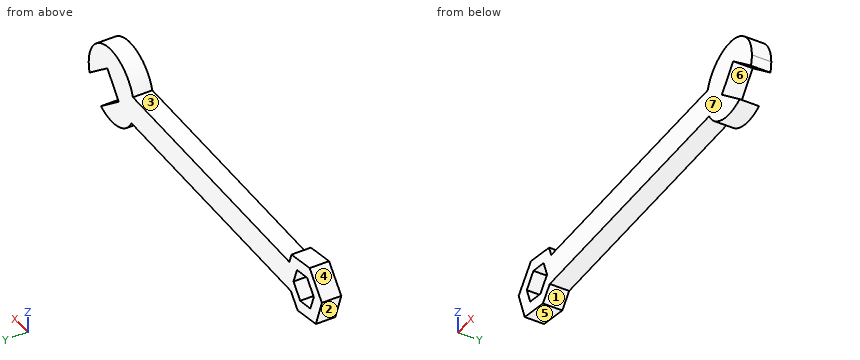
```python
from build123d import *

# Parameters (mm, degrees)
F1_DEPTH = 6.35


with BuildPart() as f1:
    # F0 (on Front) → F1 (new body)
    with BuildSketch(Plane.XZ):
        with BuildLine():
            Line((-19.535648028, 41.1698554981), (69.6690051493, 41.1698554981))
            ThreePointArc((69.6690051493, 41.1698554981), (68.2734107375, 46.0093179877), (68.8687306625, 51.0106853144))
            Line((68.8687306625, 51.0106853144), (-18.7341859771, 51.0106853144))
            Line((-18.7341859771, 51.0106853144), (-16.544501635, 44.5905560083))
            Line((-16.544501635, 44.5905560083), (-19.535648028, 41.1698554981))
        make_face()
        with BuildLine():
            ThreePointArc((68.8687306625, 51.0106853144), (68.2734107375, 46.0093179877), (69.6690051493, 41.1698554981))
            Line((69.6690051493, 41.1698554981), (76.8122168252, 41.1698554981))
            Line((76.8122168252, 41.1698554981), (76.8122168252, 44.0645504642))
            Line((76.8122168252, 44.0645504642), (76.8122168252, 51.0106853144))
            Line((76.8122168252, 51.0106853144), (68.8687306625, 51.0106853144))
        make_face()
        with BuildLine():
            Line((83.1993854847, 51.7589689942), (93.1325389176, 43.5134172284))
            ThreePointArc((93.1325389176, 43.5134172284), (93.506233567, 45.2584856945), (93.6316237892, 47.0387072915))
            ThreePointArc((93.6316237892, 47.0387072915), (82.942998604, 59.5784190647), (68.8687306625, 51.0106853144))
            Line((68.8687306625, 51.0106853144), (76.8122168252, 51.0106853144))
            Line((76.8122168252, 51.0106853144), (76.8122168252, 44.0645504642))
            Line((76.8122168252, 44.0645504642), (83.1993854847, 51.7589689942))
        make_face()
        with BuildLine():
            ThreePointArc((69.6690051493, 41.1698554981), (77.1165270466, 34.9252834632), (86.7983786546, 35.7749962091))
            Line((86.7983786546, 35.7749962091), (76.8122168252, 44.0645504642))
            Line((76.8122168252, 44.0645504642), (76.8122168252, 41.1698554981))
            Line((76.8122168252, 41.1698554981), (69.6690051493, 41.1698554981))
        make_face()
        Polygon((-24.7877831748, 41.1698554981), (-19.535648028, 41.1698554981), (-16.544501635, 44.5905560083), (-18.7341859771, 51.0106853144), (-23.0106876439, 51.0106853144), (-21.0584325376, 45.5772671147), align=None)
        Polygon((-23.3853346079, 36.7673211123), (-19.535648028, 41.1698554981), (-24.7877831748, 41.1698554981), (-30.4693889183, 42.1958620812), (-32.4216440246, 47.629280281), (-28.6922933874, 52.0366918976), (-23.0106876439, 51.0106853144), (-18.7341859771, 51.0106853144), (-19.8992053083, 54.4265085938), (-30.0947419544, 56.4392262833), (-36.9355749272, 48.6159913874), (-33.580871254, 38.7800388019), align=None)
    extrude(amount=F1_DEPTH)


solid = f1.part
```
Source: CAD feature listing. Evaluate the final solid. Frame: model axes, mm. Face numbers are marked on the shaded views. A direction names the side the tool comes from. Give positions to 0.01 mm unless a question says otherwise; leave off trailing zeros. Loops run counter-clockwise (first coordinate to the right, second up) from the corner with the lowest first, then second, coordinate; pieces in that order, holes last. Notation, with made-up numbers: (-0.5, -34.75) - (14.5, -34.75) arc R16 cw to (14.5, -7.75) - close; hole circle Ø6 at (81.25, 75.5). An arc over 180 degrees is marked (long way). Use CSV: the item, a comma, the result in double quotes. Start each with the question number.
1. Section C-C (z = 53.25). Output: boundary loops of the cut face in (x, y).
2. Section B-B (x = -26). Output: boundary loops of the cut face in (y, z).
3. Section A-A (y = -3). Output: boundary loops of the cut face in (x, z) (1 decimal), then the cut area to 3 significant figures.
4. Section D-D (x = -1.5). Output: boundary loops of the cut face in (y, z).
5. Reachability of the marked faces 1, 2 and 3 from +Z, -Z, +X, -X, +Y, -Y: full face, straight path, thin tool, end or side. Return the list, or none.
6. Pin query (flat end, axial travel): pin 1 (3 mm diameter, centred on x = 16.5, y = -2.5, fed in from +Z). Return the tip coordinate at first contact, or that it passes through.
7. Ray query, L1, parallel to X at y = -1.75, z = 49.5; L2, parallel to X at y = -2.5, z = 47.75; L3, parallel to Z at x = 30.5, y = -1. Return the intervals inside material, ascending.
8. Draft query along Z for the marked faces 4, 5, 6 and 7. Return one class per face: +Z half, -Z half, draft (parallel to the pull), parting line (faces both ways), or undercut.
Response:
1,outline,"(-32.88, -6.35) - (-19.5, -6.35) - (-19.5, 0) - (-32.88, 0) - close; (69.85, -6.35) - (92.01, -6.35) - (92.01, 0) - (69.85, 0) - close"
2,outline,"(-6.35, 37.28) - (0, 37.28) - (0, 41.39) - (-6.35, 41.39) - close; (-6.35, 51.55) - (0, 51.55) - (0, 55.63) - (-6.35, 55.63) - close"
3,outline,"(-36.9, 48.6) - (-33.6, 38.8) - (-23.4, 36.8) - (-19.5, 41.2) - (69.7, 41.2) arc R12.7 ccw to (86.8, 35.8) - (76.8, 44.1) - (83.2, 51.8) - (93.1, 43.5) arc R12.7 ccw to (68.9, 51) - (-18.7, 51) - (-19.9, 54.4) - (-30.1, 56.4) - close; hole (-32.4, 47.6) - (-30.5, 42.2) - (-24.8, 41.2) - (-21.1, 45.6) - (-23, 51) - (-28.7, 52) - close"
3,area,"1,410 mm²"
4,outline,"(-6.35, 41.17) - (0, 41.17) - (0, 51.01) - (-6.35, 51.01) - close"
5,face 1,"-Z, +Y, -Y"
5,face 2,"-Z, -X, +Y, -Y"
5,face 3,"+Z, +Y, -Y"
6,pin 1,"z = 51.01"
7,L1,"-36.16 to -30.84, -22.47 to 81.32, 85.92 to 93.39"
7,L2,"-36.64 to -32.32, -21.84 to 79.87, 88.03 to 93.61"
7,L3,"41.17 to 51.01"
8,face 4,"+Z half"
8,face 5,"-Z half"
8,face 6,"undercut"
8,face 7,"draft"
